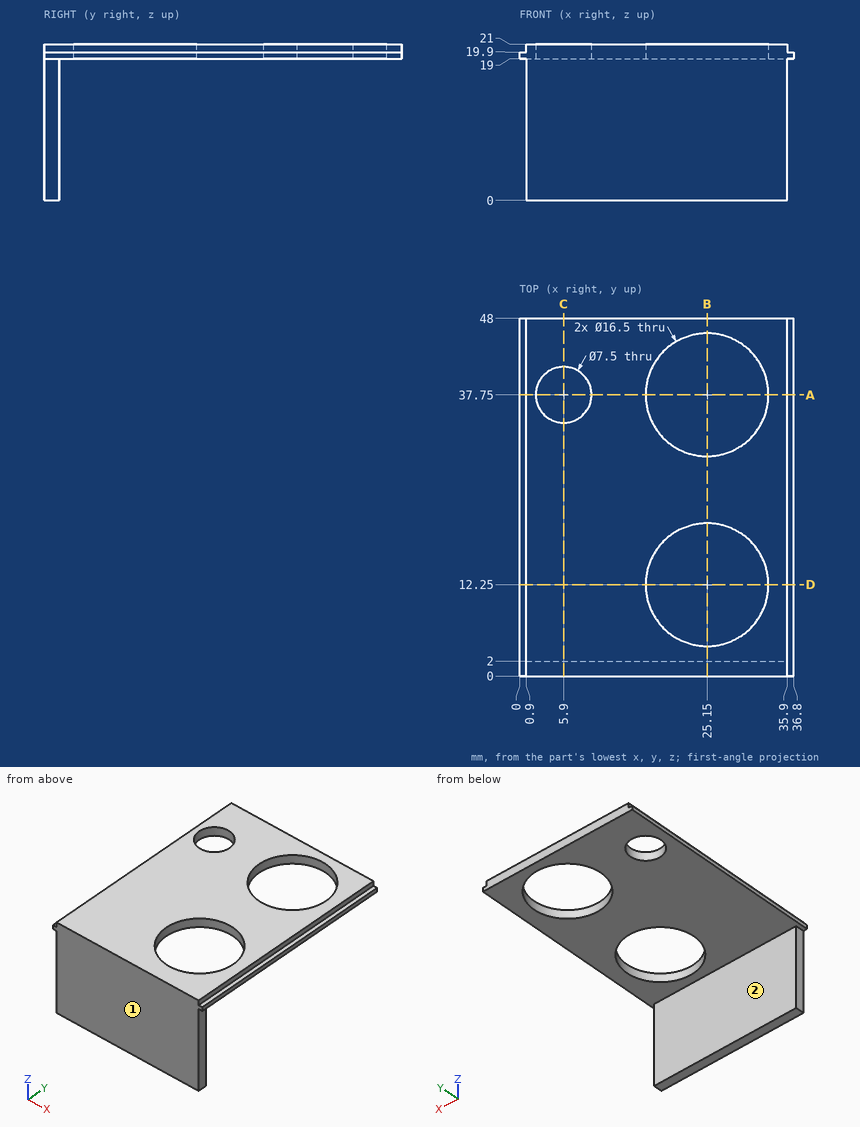
Input: dimensioned drawing with shaded views. Units: mm. Origin: part minimum x, y, z. A direction names the side the tool comes from. Round coordinates to 2 decimals unless told otherwise and drop trailing zeros. Order: outer loops, then holes, each group sorted by start corner. A loop starts at its lowest first (then second) coordinate and runs counter-clockwise, first axis right, second up. Notation, with made-up numbers: M 6.25,27 L 41.25,27 A23 ccw 41.25,65 Z; hole C 87.5,36.25 d2. An arc over 180 degrees is marked long. Use one line per item in the form item = value. Start each with the question number.
Q1. Cut plane C-C (x = 5.9). Return loops of the section in (y, z), and give its area (3 significant figures).
Q2. Cut plane B-B (x = 25.15). Return loops of the section in (y, z).
Q3. Pin query (flat end, axial travel): pin 1 Ø2 at (y, z) = (0.5, 9) entering from -X; pin 2 Ø0.6 at (y, z) = (1, 7.5) entering from +X; pin 3 Ø5.5 at (x, z) = (16.5, 11.5) entering from +Y. Return the tip coordinate at first contact, or that it passes through.
Q4. Cut plane A-A (y = 37.75). Return loops of the section in (x, z), and give its area (3 significant figures).
Q5. Cut plane D-D (y = 12.25). Return loops of the section in (x, z).
Q6. Access query for the marked faces 1 and 2. Directions: +Z, -Z, +X, -X, +Y, -Y. A direction counts if a zero-diameter tool reaches every point of the face in a straight line with its end or side. Return the directions, or none.
Q7. Material intervals for line 1 (X direction, y = 37.75, z = 20.2); line 2 (X direction, y = 37.75, z = 19.75); line 3 (Y direction, x = 25.15, z = 20.05), sorted ascending. Write a range as [from, to].
Geometry results:
q1.outline = M 0,0 L 2,0 L 2,19 L 34,19 L 34,21 L 0,21 Z; M 41.5,19 L 48,19 L 48,21 L 41.5,21 Z
q1.area = 119 mm^2
q2.outline = M 0,0 L 2,0 L 2,19 L 4,19 L 4,21 L 0,21 Z; M 20.5,19 L 29.5,19 L 29.5,21 L 20.5,21 Z; M 46,19 L 48,19 L 48,21 L 46,21 Z
q3.pin_1 = 0.9
q3.pin_2 = 35.9
q3.pin_3 = 2
q4.outline = M 0,19 L 2.15,19 L 2.15,21 L 0.9,21 L 0.9,19.9 L 0,19.9 Z; M 9.65,19 L 16.9,19 L 16.9,21 L 9.65,21 Z; M 33.4,19 L 36.8,19 L 36.8,19.9 L 35.9,19.9 L 35.9,21 L 33.4,21 Z
q4.area = 23.6 mm^2
q5.outline = M 0,19 L 16.9,19 L 16.9,21 L 0.9,21 L 0.9,19.9 L 0,19.9 Z; M 33.4,19 L 36.8,19 L 36.8,19.9 L 35.9,19.9 L 35.9,21 L 33.4,21 Z
q6.face_1 = +Z, -Z, +X, -X, -Y
q6.face_2 = -Z, +X, -X, +Y
q7.line_1 = [0.9, 2.15], [9.65, 16.9], [33.4, 35.9]
q7.line_2 = [0, 2.15], [9.65, 16.9], [33.4, 36.8]
q7.line_3 = [0, 4], [20.5, 29.5], [46, 48]
